Model file for the job. Use its own axes, mm. A direction names the side the tool comes from. Coordinates: 2 decimals unless noted, no trailing zeros. Write each loop counter-clockwise with the first axis right and the second up, starting at its lowest first coordinate (ties: lowest second). Pieces come first, ordered by that corner, then holes. Notation, with made-up numbers: M 34.25,80 L 84.25,80 A19 ccw 84.25,84 Z; hole C 28,78 d4. An arc over 180 degrees is marked long. Put each result on its own line as item: value. Start each with the question number.
Q1. Cut at A-A (x = 278.5). Write the cut outline in (y, z).
Q2. Drill centre lines: line 1 along X through (y, z) = (4.75, -5.5); line 2 along X through (y, z) = (3.75, 4.25); line 3 along Z through (x, y) = (375, -4.5). Where is each one in solid material? Low to high.
Q3. Which spindle directions (+Z, -Z, +X, -X, +Y, -Y) get a long thin tool onto all of the face, cutting with end or side? Do faces 1 (the flat face through (665, 5.1, 1.2)), 2 (the flat face through (12, -3, 5)), 3 (the flat face through (675, -7, 0)). Say none if no direction does.
Q4. Pull direction X, two halves, no side cores. Call faces 4 (the cylindrical face through (689.942, -5.723, -1.802)), 5 (the flat face through (705, -4, -4)), 6 (the flat face through (660, 2, 5)): pulls with the +X half, pulls with the -X half, needs draft (parallel to the pull), parting line crosses it, or undercut.
Q5. Drop flat-ended pins along their axis: pin 1 (1.5 mm diameter, centred on x = 521, y = -3, fed in from -Z); pin 2 (4 mm diameter, centred on x = 667.5, y = 2, fed in from -Z); pin 3 (2.5 mm diameter, centred on x = 666.5, y = -1, fed in from +Z). Give the stop position or say it passes through.
```python
from build123d import *

# Parameters (mm, degrees)
FILLET1_R          = 0.3
CHAMFER1_SIZE      = 0.5
CHAMFER2_SIZE      = 0.2
CUT_EXTRUDE1_DEPTH = 5


with BuildPart() as part:
    # Sketch1 → Revolve1 (revolve)
    with BuildSketch(Plane.XY, mode=Mode.PRIVATE) as revolve1_sk:
        Polygon((675, 7.5), (665, 7.5), (665, 5), (660, 5), (660, 7.5), (12, 7.5), (12, 5), (4, 5), (4, 4.8), (2.85, 4.8), (2.85, 5), (0, 5), (0, 0), (720, 0), (720, 5), (705, 5), (705, 6), (675, 6), align=None)
    revolve(revolve1_sk.sketch.rotate(Axis((0, 0, 0), (1, 0, 0)), 180), axis=Axis((0, 0, 0), (1, 0, 0)))

    # Fillet1
    fillet1_edges = [part.edges().sort_by_distance(p)[0] for p in [
        (675, 6, 0),
        (12, 5, 0),
    ]]
    fillet(fillet1_edges, radius=FILLET1_R)

    # Chamfer1
    chamfer1_edges = [part.edges().sort_by_distance(p)[0] for p in [
        (720, 5, 0),
        (0, 5, 0),
    ]]
    chamfer(chamfer1_edges, length=CHAMFER1_SIZE)

    # Chamfer2
    chamfer2_edges = [part.edges().sort_by_distance(p)[0] for p in [
        (675, 7.5, 0),
    ]]
    chamfer(chamfer2_edges, length=CHAMFER2_SIZE)

    # Sketch2 → Cut-Extrude1 (cut)
    with BuildSketch(Plane.ZY.offset(-665)):
        with BuildLine():
            Line((-6, 4.5), (-6, -4.5))
            ThreePointArc((-6, -4.5), (-7.5, 0), (-6, 4.5))
        make_face()
        with BuildLine():
            Line((6, 4.5), (6, -4.5))
            ThreePointArc((6, -4.5), (7.5, 0), (6, 4.5))
        make_face()
    extrude(amount=-CUT_EXTRUDE1_DEPTH, mode=Mode.SUBTRACT)


solid = part.part
```
Computed values:
1. outline: C 0,0 d15
2. line 1: 12 to 660, 665 to 675
2. line 2: 12 to 660, 665 to 705
2. line 3: -6 to 6
3. face 1: none
3. face 2: -X
3. face 3: +X
4. face 4: needs draft
4. face 5: pulls with the +X half
4. face 6: undercut
5. pin 1: z = -7.15
5. pin 2: z = -6
5. pin 3: z = 6
